```python
from build123d import *

# Parameters (mm, degrees)
SKETCH_1_R               = 11
EXTRUDE_1_DEPTH          = 2.2
SKETCH_2_R               = 5
EXTRUDE_2_DEPTH          = 10
SKETCH_3_R               = 1.5
CUT_EXTRUDE_1_DEPTH      = 10
CUT_EXTRUDE_2_DEPTH      = 10
CUT_EXTRUDE_2_DEPTH_BACK = 10
SKETCH_4_R               = 1.6
SKETCH_5_R               = 2.5
CUT_EXTRUDE_3_DEPTH      = 50


with BuildPart() as part:
    # Sketch 1 → Extrude 1 (new body)
    with BuildSketch(Plane.XY):
        Circle(SKETCH_1_R)
    extrude(amount=EXTRUDE_1_DEPTH)

    # Sketch 2 → Extrude 2 (add)
    with BuildSketch(Plane.XY.offset(2.2)):
        Circle(SKETCH_2_R)
    extrude(amount=EXTRUDE_2_DEPTH)

    # Sketch 3 → Cut-Extrude 1 (cut)
    with BuildSketch(Plane.XY.offset(2.2)):
        with Locations((8, 0)):
            Circle(SKETCH_3_R)
        with Locations((0, -8)):
            Circle(SKETCH_3_R)
        with Locations((-8, 0)):
            Circle(SKETCH_3_R)
        with Locations((0, 8)):
            Circle(SKETCH_3_R)
    extrude(amount=-CUT_EXTRUDE_1_DEPTH, mode=Mode.SUBTRACT)

    # Sketch 4 → Cut-Extrude 2 (cut, two sides: drawn at the far end of the back side and taken through both)
    with BuildSketch(Plane(origin=(0, 0, 0), x_dir=(0, 0, -1), z_dir=(1, 0, 0)).offset(-CUT_EXTRUDE_2_DEPTH_BACK)):
        with Locations(Location((-6.2, 0, 0), (0, 0, 180))):
            Circle(SKETCH_4_R)
    extrude(amount=CUT_EXTRUDE_2_DEPTH + CUT_EXTRUDE_2_DEPTH_BACK, mode=Mode.SUBTRACT)

    # Sketch 5 → Cut-Extrude 3 (cut)
    with BuildSketch(Plane(origin=(0, 0, 0), x_dir=(-1, 0, 0), z_dir=(0, 0, -1))):
        Circle(SKETCH_5_R)
    extrude(amount=-CUT_EXTRUDE_3_DEPTH, mode=Mode.SUBTRACT)


solid = part.part
```
CAD build for the part. Positions are in the model's coordinates, mm. A direction names the side the tool comes from. Round coordinates to 2 decimals unless told otherwise and drop trailing zeros. Order: outer loops, then holes, each group sorted by start corner. A loop starts at its lowest first (then second) coordinate and runs counter-clockwise, first axis right, second up. Notation, with made-up numbers: (-26, -2) -> (16, -2) arc R38 cw to (16, 37) -> close; hole circle Ø1 at (38.25, -17). An arc over 180 degrees is marked (long way). Write item = value, one per line.
(1) Flat gauge pins, fed straight in: P1, Ø5, axis at x = 2, z = 6, coming from the -Y side; P2, Ø8, axis at x = -8, y = -7.5, coming from the +Z side; P3, Ø5, axis at y = 0, z = 6.2, coming from the +X side. Where does each tip first touch, or does it go through?
Answers follow:
P1 = -5
P2 = 2.2
P3 = 5
(2) Drill centre lines: L1, parallel to Y at x = 0, z = 1.05; L2, parallel to Y at x = 0, z = 5.25; L3, parallel to Z at x = -3.5, y = -4.5. Where is each one in solid material? Low to high.
Answers follow:
L1 = -11 to -9.5, -6.5 to -2.5, 2.5 to 6.5, 9.5 to 11
L2 = -5 to -2.5, 2.5 to 5
L3 = 0 to 2.2
(3) Cut at D-D (y = -8). Write the cut outline in (x, z), plus the area to 3 significant figures.
Answers follow:
outline = (-7.55, 0) -> (-1.5, 0) -> (-1.5, 2.2) -> (-7.55, 2.2) -> close; (1.5, 0) -> (7.55, 0) -> (7.55, 2.2) -> (1.5, 2.2) -> close
area = 26.6 mm²
(4) 3-axis set-ups, long thin cutter, end or side, ignore diameter. For faces 4 (the cylindrical face through (4.619, -1.915, 7.13)), 5 (the cylindrical face through (-0.325, 6.536, 1.115)): which of +Z, -Z, +X, -X, +Y, -Y reach the whole face in a straight line?
Answers follow:
face_4 = +Z
face_5 = +Z, -Z
(5) Cut at C-C (z = 5.5). Write the cut outline in (x, y).
Answers follow:
outline = (-4.79, -1.44) arc R5 ccw to (4.79, -1.44) -> (2.04, -1.44) arc R2.5 cw to (-2.04, -1.44) -> close; (-4.79, 1.44) -> (-2.04, 1.44) arc R2.5 cw to (2.04, 1.44) -> (4.79, 1.44) arc R5 ccw to start
(6) Pull direction Y, two halves, no side cores. Call faces 1 (the cylindrical face through (-2.38, -10.74, 1.08)), 2 (the cylindrical face through (6.5, 0.07, 1.12)), 3 (the flat face through (0, 3, 0)): +Y half, -Y half, draft (parallel to the pull), parting line (faces both ways), or undercut.
Answers follow:
face_1 = parting line
face_2 = undercut
face_3 = draft
(7) Cut at A-A (y = 0). Write the cut outline in (x, z), plus the area to 3 significant figures.
Answers follow:
outline = (-11, 0) -> (-9.5, 0) -> (-9.5, 2.2) -> (-11, 2.2) -> close; (-6.5, 0) -> (-2.5, 0) -> (-2.5, 4.6) -> (-5, 4.6) -> (-5, 2.2) -> (-6.5, 2.2) -> close; (-5, 7.8) -> (-2.5, 7.8) -> (-2.5, 12.2) -> (-5, 12.2) -> close; (2.5, 0) -> (6.5, 0) -> (6.5, 2.2) -> (5, 2.2) -> (5, 4.6) -> (2.5, 4.6) -> close; (2.5, 7.8) -> (5, 7.8) -> (5, 12.2) -> (2.5, 12.2) -> close; (9.5, 0) -> (11, 0) -> (11, 2.2) -> (9.5, 2.2) -> close
area = 58.2 mm²
(8) Cut at B-B (x = 0). Write the cut outline in (y, z), plus the area to 3 significant figures.
Answers follow:
outline = (-11, 0) -> (-9.5, 0) -> (-9.5, 2.2) -> (-11, 2.2) -> close; (-6.5, 0) -> (-2.5, 0) -> (-2.5, 12.2) -> (-5, 12.2) -> (-5, 2.2) -> (-6.5, 2.2) -> close; (2.5, 0) -> (6.5, 0) -> (6.5, 2.2) -> (5, 2.2) -> (5, 12.2) -> (2.5, 12.2) -> close; (9.5, 0) -> (11, 0) -> (11, 2.2) -> (9.5, 2.2) -> close
area = 74.2 mm²
